Part model, mm, in its own coordinate system. Face numbers are marked on the shaded views. Give positions to 0.01 mm unless a question says otherwise; leave off trailing zeros. Order: outer loops, then holes, each group sorted by start corner. A loop starts at its lowest first (then second) coordinate and runs counter-clockwise, first axis right, second up.
1. Mould opens along X. For the marked faces 1, 2, 3 and 4 say: +X half, -X half, draft (parallel to the pull), parting line (faces both ways), or undercut.
2. Slice it at A-A on y = -3. List the corners of the cut face in (x, z).
3. Drop flat-ended pins along their axis: pin 1 Ø3 at (x, z) = (-4, 7.5) entering from -Y; pin 2 Ø4 at (y, z) = (-5.5, 1.5) entering from +X; pin 3 Ø6.5 at (x, z) = (-10.11, 0) entering from +Y; pin 4 Ø1 at (y, z) = (-1, -6) entering from -X. Give the stop position or say it passes through.
4. Probe line 1 (X direction, y = -5, z = 0); line 2 (X direction, y = 1.2, z = 0); line 3 (Y direction, x = -18, z = -11). List the from-to ranges inside material, lowest first.
from build123d import *

# Parameters (mm, degrees)
SKETCH1_R           = 3.65
BOSS_EXTRUDE1_DEPTH = 5
SKETCH_1_R          = 5.65
SKETCH_1_R_2        = 3.65
EXTRUDE_1_DEPTH     = 7.5
EXTRUDE_2_DEPTH     = 5


with BuildPart() as part:
    # Sketch1 → Boss-Extrude1 (new body)
    with BuildSketch(Plane(origin=(0, 4, 0), x_dir=(1, 0, 0), z_dir=(0, 1, 0))):
        with BuildLine():
            Line((1.43808022, 3.600125745), (2.081641936, 4))
            ThreePointArc((2.081641936, 4), (2.861028333, 4.588201733), (3.521749436, 5.30713988))
            ThreePointArc((3.521749436, 5.30713988), (3.405395609, 5.596745198), (3.282888305, 5.883801663))
            ThreePointArc((3.282888305, 5.883801663), (1.93527598, 5.894040025), (0.627094961, 5.57027124))
            ThreePointArc((0.627094961, 5.57027124), (0.366286148, 6.046375), (0.084372603, 6.510293938))
            ThreePointArc((0.084372603, 6.510293938), (1.018855105, 7.48132754), (1.683794586, 8.65351323))
            ThreePointArc((1.683794586, 8.65351323), (1.496450048, 8.903135899), (1.303821399, 9.148703928))
            ThreePointArc((1.303821399, 9.148703928), (-0.000522033, 8.809805691), (-1.180330337, 8.158486898))
            ThreePointArc((-1.180330337, 8.158486898), (-1.555477026, 8.550865528), (-1.947855656, 8.926012217))
            ThreePointArc((-1.947855656, 8.926012217), (-1.296536862, 10.105820521), (-0.957638625, 11.410163953))
            ThreePointArc((-0.957638625, 11.410163953), (-1.203206655, 11.602792602), (-1.452829324, 11.79013714))
            ThreePointArc((-1.452829324, 11.79013714), (-2.625015014, 11.125197659), (-3.596048616, 10.190715157))
            ThreePointArc((-3.596048616, 10.190715157), (-4.059967554, 10.472628702), (-4.536071314, 10.733437515))
            ThreePointArc((-4.536071314, 10.733437515), (-4.212302529, 12.041618533), (-4.222540891, 13.389230859))
            ThreePointArc((-4.222540891, 13.389230859), (-4.509597355, 13.511738163), (-4.799202674, 13.62809199))
            ThreePointArc((-4.799202674, 13.62809199), (-5.759348103, 12.682425791), (-6.455432668, 11.528463019))
            ThreePointArc((-6.455432668, 11.528463019), (-6.976508546, 11.680699536), (-7.503891752, 11.809396783))
            ThreePointArc((-7.503891752, 11.809396783), (-7.529737283, 13.156800143), (-7.888414517, 14.455843809))
            ThreePointArc((-7.888414517, 14.455843809), (-8.197396993, 14.499881098), (-8.507248835, 14.537314892))
            ThreePointArc((-8.507248835, 14.537314892), (-9.18992168, 13.375367565), (-9.563620196, 12.080565177))
            ThreePointArc((-9.563620196, 12.080565177), (-10.106342554, 12.09275), (-10.649064912, 12.080565177))
            ThreePointArc((-10.649064912, 12.080565177), (-11.022763428, 13.375367565), (-11.705436272, 14.537314892))
            ThreePointArc((-11.705436272, 14.537314892), (-12.015288115, 14.499881098), (-12.324270591, 14.455843809))
            ThreePointArc((-12.324270591, 14.455843809), (-12.682947825, 13.156800143), (-12.708793355, 11.809396783))
            ThreePointArc((-12.708793355, 11.809396783), (-13.236176561, 11.680699536), (-13.757252439, 11.528463019))
            ThreePointArc((-13.757252439, 11.528463019), (-14.453337005, 12.682425791), (-15.413482434, 13.62809199))
            ThreePointArc((-15.413482434, 13.62809199), (-15.703087752, 13.511738163), (-15.990144217, 13.389230859))
            ThreePointArc((-15.990144217, 13.389230859), (-16.000382579, 12.041618533), (-15.676613793, 10.733437515))
            ThreePointArc((-15.676613793, 10.733437515), (-16.152717554, 10.472628702), (-16.616636492, 10.190715157))
            ThreePointArc((-16.616636492, 10.190715157), (-17.587670094, 11.125197659), (-18.759855783, 11.79013714))
            ThreePointArc((-18.759855783, 11.79013714), (-19.009478453, 11.602792602), (-19.255046482, 11.410163953))
            ThreePointArc((-19.255046482, 11.410163953), (-18.916148245, 10.105820521), (-18.264829452, 8.926012217))
            ThreePointArc((-18.264829452, 8.926012217), (-18.657208082, 8.550865528), (-19.032354771, 8.158486898))
            ThreePointArc((-19.032354771, 8.158486898), (-20.212163074, 8.809805691), (-21.516506507, 9.148703928))
            ThreePointArc((-21.516506507, 9.148703928), (-21.709135156, 8.903135899), (-21.896479694, 8.65351323))
            ThreePointArc((-21.896479694, 8.65351323), (-21.231540213, 7.48132754), (-20.297057711, 6.510293938))
            ThreePointArc((-20.297057711, 6.510293938), (-20.578971255, 6.046375), (-20.839780068, 5.57027124))
            ThreePointArc((-20.839780068, 5.57027124), (-22.147961087, 5.894040025), (-23.495573413, 5.883801663))
            ThreePointArc((-23.495573413, 5.883801663), (-23.618080717, 5.596745198), (-23.734434544, 5.30713988))
            ThreePointArc((-23.734434544, 5.30713988), (-22.788768345, 4.346994451), (-21.634805572, 3.650909885))
            ThreePointArc((-21.634805572, 3.650909885), (-21.803584999, 3.067429176), (-21.942853375, 2.47620963))
            ThreePointArc((-21.942853375, 2.47620963), (-22.095637401, -1.578420611), (-20.898643838, -5.455349261))
            ThreePointArc((-20.898643838, -5.455349261), (-7.038913378, -11.697242445), (1.974222624, 0.542722358))
            ThreePointArc((1.974222624, 0.542722358), (3.269025011, 0.916420874), (4.430972339, 1.599093719))
            ThreePointArc((4.430972339, 1.599093719), (4.393538544, 1.908945561), (4.349501255, 2.217928037))
            ThreePointArc((4.349501255, 2.217928037), (3.050457589, 2.576605271), (1.70305423, 2.602450802))
            ThreePointArc((1.70305423, 2.602450802), (1.581217534, 3.104116905), (1.43808022, 3.600125745))
        make_face()
        with Locations(Location((-10.106342554, 0, 0), (0, 0, 90))):
            Circle(SKETCH1_R, mode=Mode.SUBTRACT)
    extrude(amount=-BOSS_EXTRUDE1_DEPTH)

    # 草图1 → 凸台-拉伸1 (add)
    with BuildSketch(Plane.XZ.offset(1)):
        with Locations(Location((-10.106342554, 0, 0), (0, 0, 90))):
            Circle(SKETCH_1_R)
        with Locations(Location((-10.106342554, 0, 0), (0, 0, 270))):
            Circle(SKETCH_1_R_2, mode=Mode.SUBTRACT)
    extrude(amount=EXTRUDE_1_DEPTH)

    # 草图2 → 凸台-拉伸2 (add)
    with BuildSketch(Plane(origin=(0, 4, 0), x_dir=(1, 0, 0), z_dir=(0, 1, 0))):
        with BuildLine():
            Line((-20.290866754, -11.657484407), (-16.715112634, -10.127129929))
            Line((-16.715112634, -10.127129929), (-22.184948493, 0.584706011))
            Line((-22.184948493, 0.584706011), (-30.168856615, -2.832254199))
            ThreePointArc((-30.168856615, -2.832254199), (-41.120771134, -18.396815496), (-59.941897602, -15.574547178))
            Line((-59.941897602, -15.574547178), (-71.283909207, -20.428711551))
            ThreePointArc((-71.283909207, -20.428711551), (-43.218414154, -30.97827059), (-20.290866754, -11.657484407))
        make_face()
    extrude(amount=-EXTRUDE_2_DEPTH)

    # 草图3 → 切除-旋转1 (revolve, cut)
    with BuildSketch(Plane(origin=(-18.284564858, 0, -22.548473972), x_dir=(0.7767217347580433, 0, -0.6298439066581941), z_dir=(0.6298439066581941, 0, 0.7767217347580433))):
        Polygon((-60.074661111, 4), (-56.274661111, -1.234092457), (-56.274661111, 4), align=None)
    revolve(axis=Axis((-48.246342554, -1, 1.74754128), (0, 1, 0)), mode=Mode.SUBTRACT)


solid = part.part
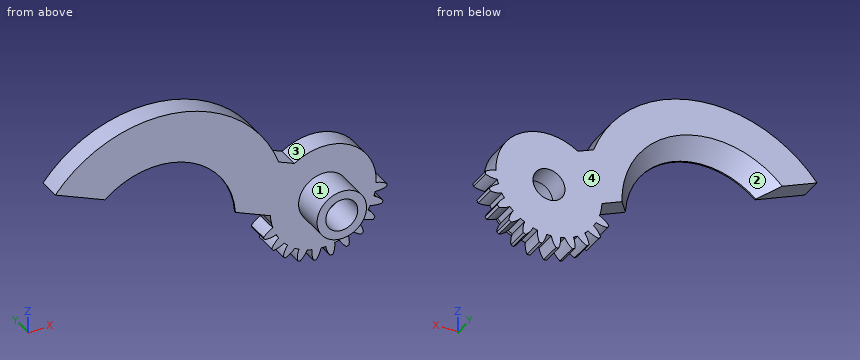
Data:
1. face 1: parting line
1. face 2: undercut
1. face 3: undercut
1. face 4: draft
2. outline: circle Ø11.3 at (-10.11, 0); hole circle Ø7.3 at (-10.11, 0)
3. pin 1: stops at y = -1
3. pin 2: stops at x = -4.46
3. pin 3: passes through
3. pin 4: stops at x = -23.66
4. line 1: x = -15.76 to -13.76, -6.46 to -4.46
4. line 2: x = -23.55 to -13.76, -6.46 to 1.99
4. line 3: y = -1 to 4
